```python
from build123d import *

# Parameters (mm, degrees)
F0_R     = 72.5682102396
F1_DEPTH = 20


with BuildPart() as f1:
    # F0 (on Top) → F1 (new body)
    with BuildSketch(Plane.XY):
        Circle(F0_R)
        with BuildLine():
            ThreePointArc((22.1639949501, -24.0462341013), (35.0578120406, -24.024439202), (33.1385050428, -36.7746256645))
            add(Edge.make_bspline(
                [(-26.8195513636, -50.0101186335), (-16.3397293577, -50.3620265328), (2.2569416099, -51.0958463241), (19.6306451708, -46.8878952171), (29.1549246758, -40.8179573715), (33.1385050428, -36.7746256645)],
                knots=[0, 0, 0, 0, 0.3979017019, 0.7032152945, 1, 1, 1, 1], degree=3))
            Line((-26.8195513636, -50.0101186335), (-6.967373221, 45.1261032148))
            ThreePointArc((-6.967373221, 45.1261032148), (-6.8654000382, 45.7190077179), (-6.7217441894, 46.303214254))
            ThreePointArc((-6.7217441894, 46.303214254), (3.8794477521, 52.1297184336), (9.5709745897, 41.4554529416))
            Line((9.5709745897, 41.4554529416), (6.8737706169, 29.0141291916))
            Line((6.8737706169, 29.0141291916), (17.6235703774, 28.8198585581))
            ThreePointArc((17.6235703774, 28.8198585581), (26.5673663066, 19.7578688539), (16.4828933265, 11.9851892814))
            Line((16.4828933265, 11.9851892814), (3.4721444827, 11.9851892814))
            Line((3.4721444827, 11.9851892814), (-5.8604949154, -32.8977927566))
            add(Edge.make_bspline(
                [(-5.8604949154, -32.8977927566), (-0.251077846, -32.8079528339), (10.9390044639, -32.2469206836), (17.7138596773, -27.5571513921), (22.1639949501, -24.0462341013)],
                knots=[0, 0, 0, 0, 0.5182413567, 1, 1, 1, 1], degree=3))
        make_face(mode=Mode.SUBTRACT)
    extrude(amount=F1_DEPTH)


solid = f1.part
```
Input: part model. Units: mm. Frame: model coordinates. A direction names the side the tool comes from. Coordinates: 2 decimals unless noted, no trailing zeros. Loops run counter-clockwise (first coordinate to the right, second up) from the corner with the lowest first, then second, coordinate; pieces in that order, holes last. Notation, with made-up numbers: M 8,9.25 L 37,9.25 A24 ccw 37,31.25 Z; hole C 44,34.25 d1. An arc over 180 degrees is marked long. One line per item, written item: value.
(1) Line query: line 1 along X through (y, z) = (-27.5, 13.5); line 2 along Y through (x, z) = (14.5, 5.5) (3 decimals); line 3 along X through (y, z) = (50, 3.25). Output: solid intervals per line, ascending. Write a range as from..to.
Filled in:
line 1: -67.16..-22.12, -4.74..17.52, 36.86..67.16
line 2: -71.105..-47.799, -29.325..11.985, 28.876..71.105
line 3: -52.59..-4.55, 7.46..52.59
(2) Pin query (flat end, axial travel): pin 1 (22 mm diameter, centred on x = 18.09, y = 20.33, fed in from +Z); pin 2 (2 mm diameter, centred on y = 40.5, z = 18, fed in from +X); pin 3 (10 mm diameter, centred on y = 19.5, z = 10, fed in from +X); pin 4 (2 mm diameter, centred on x = -6.5, z = 11.5, fed in from +Y). Return the tip coordinate at first contact, or that it passes through.
Filled in:
pin 1: z = 20
pin 2: x = 60.88
pin 3: x = 71.1
pin 4: y = 72.36
(3) Section C-C (y = 56). Output: boundary loops of the cut face in (x, z), and give its area (3 significant figures).
Filled in:
outline: M -46.15,0 L 46.15,0 L 46.15,20 L -46.15,20 Z
area: 1,850 mm^2
(4) Pull-direction query (Y, two-part tool) for faces 1 (the flat face through (15, 1, 20)), 2 (the flat face through (8.24, 35.32, 9.86)), 3 (the cylindrical face through (33.49, -64.38, 9.86)); classes: +Y half, -Y half, draft (parallel to the pull), parting line (faces both ways), or undercut.
Filled in:
face 1: draft
face 2: undercut
face 3: parting line
(5) Reachability of faces 4 (the flat face through (15, 1, 0)), 5 (the flat face through (10, 11.985, 10)) from +Z, -Z, +X, -X, +Y, -Y: full face, straight path, thin tool, end or side. Return the list, or none.
Filled in:
face 4: -Z, +X, -X, +Y, -Y
face 5: +Z, -Z
(6) Section A-A (y = 0). Output: boundary loops of the cut face in (x, z), and give its area (3 significant figures).
Filled in:
outline: M -72.57,0 L -16.38,0 L -16.38,20 L -72.57,20 Z; M 0.98,0 L 72.57,0 L 72.57,20 L 0.98,20 Z
area: 2,560 mm^2
(7) Section B-B (x = 0). Give the number of separate pieces and of enclosed holes in the cut face, and give its area (3 significant figures).
Filled in:
separate pieces: 3
enclosed holes: 0
area: 1,410 mm^2
